Design review of the part built by this model. Coordinates are the model's own, in mm. Round coordinates to 2 decimals unless told otherwise and drop trailing zeros. Order: outer loops, then holes, each group sorted by start corner. A loop starts at its lowest first (then second) coordinate and runs counter-clockwise, first axis right, second up. Notation, with made-up numbers: M 48.5,-3.75 L 77.5,-3.75 A11 cw 77.5,11.25 Z; hole C 46.25,57.5 d7. An arc over 180 degrees is marked long. Write each question's results on one line, items separated by ' | '. Start each with the question number.
Item 1: Wall thickness on line 1 (Z direction, x = -16, y = 3.5); line 2 (Z direction, x = -19.5, y = 0.45); line 3 (X direction, y = 2.7, z = -26): over which ranges is each line inside the solid? List them lowest first. Write a range as [from, to].
Item 2: Take a section at B-B, the plane y = 1.4. Write out the cut boundary in (x, z), plus the area to 3 significant figures.
Item 3: Take a section at D-D, the plane z = -92. Write out the cut boundary in (x, y), plus the area to 3 significant figures.
Item 4: Take a section at C-C, the plane x = -11.25. Write out the cut boundary in (y, z), plus the area to 3 significant figures.
Item 5: Clearance check with flat-ended pins moving along their axes: pin 1 (12 mm diameter, centred on x = -24, z = -78, fed in from -Y); pin 2 (1 mm diameter, centred on y = 3, z = -45.5, fed in from -X); pin 3 (1.5 mm diameter, centred on x = -13.5, y = 2.5, fed in from -Z). State where each tip first meets the part, or that it passes through.
Item 6: Take a section at A-A, the plane z = -72. Write out the cut boundary in (x, y), plus the area to 3 significant figures.
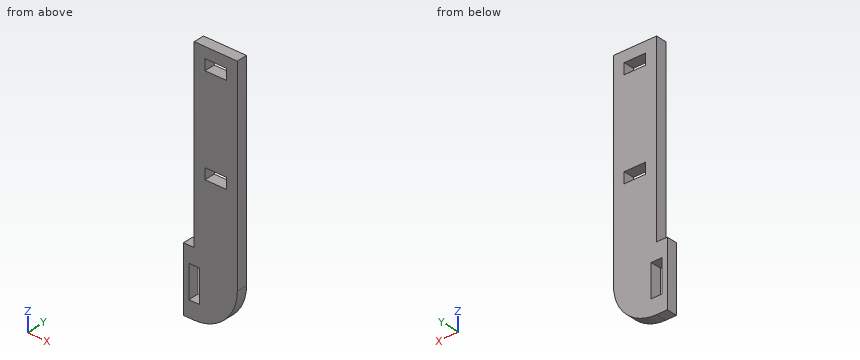
```python
from build123d import *

# Parameters (mm, degrees)
SKETCH1_W           = 10
SKETCH1_H           = 5
SKETCH1_W_2         = 5
SKETCH1_H_2         = 15
BOSS_EXTRUDE1_DEPTH = 5


with BuildPart() as part:
    # Sketch1 → Boss-Extrude1 (new body)
    with BuildSketch(Plane(origin=(0, 0, 0), x_dir=(1, 0, 0), z_dir=(0, 1, 0))):
        with BuildLine():
            Line((-25.064538889, 20.027213551), (-5.064538889, 20.027213551))
            Line((-5.064538889, 20.027213551), (-5.064538889, 80.027213551))
            Line((-5.064538889, 80.027213551), (-5.064538889, 115.027213551))
            ThreePointArc((-5.064538889, 115.027213551), (-10.922403265, 129.169349175), (-25.064538889, 135.027213551))
            Line((-25.064538889, 135.027213551), (-30.064538889, 135.027213551))
            Line((-30.064538889, 135.027213551), (-30.064538889, 105.027213551))
            Line((-30.064538889, 105.027213551), (-25.064538889, 105.027213551))
            Line((-25.064538889, 105.027213551), (-25.064538889, 80.027213551))
            Line((-25.064538889, 80.027213551), (-25.064538889, 20.027213551))
        make_face()
        with Locations((-15.064538889, 27.527213551)):
            Rectangle(SKETCH1_W, SKETCH1_H, mode=Mode.SUBTRACT)
        with Locations((-15.064538889, 72.527213551)):
            Rectangle(SKETCH1_W, SKETCH1_H, mode=Mode.SUBTRACT)
        with Locations((-25.064538889, 120.027213551)):
            Rectangle(SKETCH1_W_2, SKETCH1_H_2, mode=Mode.SUBTRACT)
    extrude(amount=BOSS_EXTRUDE1_DEPTH)


solid = part.part
```
Results list:
1) line 1: [-132.86, -75.03], [-70.03, -30.03], [-25.03, -20.03] | line 2: [-134.24, -75.03], [-70.03, -30.03], [-25.03, -20.03] | line 3: [-25.06, -20.06], [-10.06, -5.06]
2) outline: M -30.06,-135.03 L -25.06,-135.03 A20 ccw -5.06,-115.03 L -5.06,-20.03 L -25.06,-20.03 L -25.06,-105.03 L -30.06,-105.03 Z; hole M -27.56,-127.53 L -22.56,-127.53 L -22.56,-112.53 L -27.56,-112.53 Z; hole M -20.06,-75.03 L -10.06,-75.03 L -10.06,-70.03 L -20.06,-70.03 Z; hole M -20.06,-30.03 L -10.06,-30.03 L -10.06,-25.03 L -20.06,-25.03 Z | area: 2,190 mm²
3) outline: M -25.06,0 L -5.06,0 L -5.06,5 L -25.06,5 Z | area: 100 mm²
4) outline: M 0,-129.49 L 5,-129.49 L 5,-75.03 L 0,-75.03 Z; M 0,-70.03 L 5,-70.03 L 5,-30.03 L 0,-30.03 Z; M 0,-25.03 L 5,-25.03 L 5,-20.03 L 0,-20.03 Z | area: 497 mm²
5) pin 1: y = 0 | pin 2: x = -25.06 | pin 3: z = -131.85
6) outline: M -25.06,0 L -20.06,0 L -20.06,5 L -25.06,5 Z; M -10.06,0 L -5.06,0 L -5.06,5 L -10.06,5 Z | area: 50.0 mm²
